Could you check a few things on this model? Use its own coordinates, in mm. Coordinates: 2 decimals unless noted, no trailing zeros. Loops run counter-clockwise (first coordinate to the right, second up) from the corner with the lowest first, then second, coordinate; pieces in that order, holes last.
1) Imagine slicing it at A-A on y = -1. Please give me the cut outline in (x, z).
2) Will these pins go through, and if not, where does the flat tip stop? P1, Ø1, axis at x = -28, y = -2.5, coming from the +Z side; P2, Ø1.5, axis at y = -1.5, z = 35.5, coming from the -X side; P3, Ø1, axis at x = -58.5, y = -1, coming from the +Z side.
3) Imagine slicing it at B-B on x = 12.5. Please give me the cut outline in (y, z).
4) If I drill on line 1 along X through (y, z) = (-2.7, 20); line 2 along Z through (x, y) = (19.5, -0.3); line 3 along X through (y, z) = (-2.1, 27.5), over which ranges is the centre line in solid material (lowest first)?
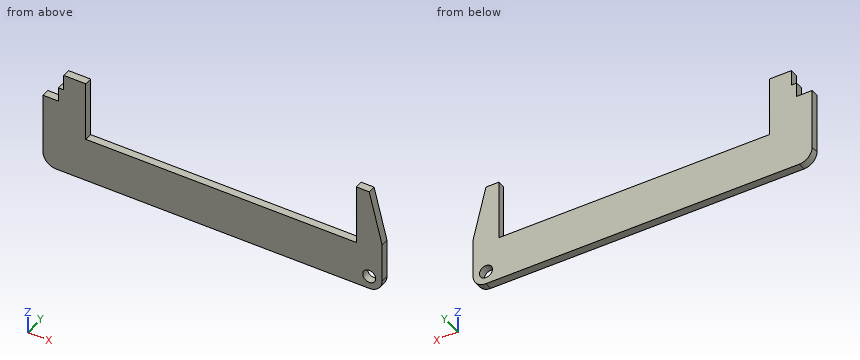
```python
from build123d import *

# Parameters (mm, degrees)
F0_R     = 2.5
F1_DEPTH = 3
F2_W     = 2
F2_H     = 6
F3_DEPTH = 3.001


with BuildPart() as f1:
    # F0 (on Front) → F1 (new body)
    with BuildSketch(Plane.XZ):
        with BuildLine():
            Line((-59.771481, 28.5), (-65.771481, 28.5))
            Line((-65.771481, 28.5), (-65.771481, 5))
            ThreePointArc((-65.771481, 5), (-64.307015, 1.464466), (-60.771481, 0))
            Line((-60.771481, 0), (60.228519, 0))
            ThreePointArc((60.228519, 0), (63.764053, 1.464466), (65.228519, 5))
            Line((65.228519, 5), (65.228519, 20))
            Line((65.228519, 20), (60.228519, 40))
            Line((60.228519, 40), (55.228519, 40))
            Line((55.228519, 40), (55.228519, 17))
            Line((55.228519, 17), (-49.271481, 17))
            Line((-49.271481, 17), (-49.271481, 40))
            Line((-49.271481, 40), (-59.771481, 40))
            Line((-59.771481, 40), (-59.771481, 28.5))
        make_face()
        with Locations((60.228519, 5)):
            Circle(F0_R, mode=Mode.SUBTRACT)
    extrude(amount=F1_DEPTH)

    # F2 (on face) → F3 (cut, through all)
    with BuildSketch(Plane.XZ.offset(3)):
        with Locations((-58.771481, 37)):
            Rectangle(F2_W, F2_H)
    extrude(amount=-F3_DEPTH, mode=Mode.SUBTRACT)


solid = f1.part
```
Filled in:
1. outline: (-65.77, 5) arc R5 ccw to (-60.77, 0) - (60.23, 0) arc R5 ccw to (65.23, 5) - (65.23, 20) - (60.23, 40) - (55.23, 40) - (55.23, 17) - (-49.27, 17) - (-49.27, 40) - (-57.77, 40) - (-57.77, 34) - (-59.77, 34) - (-59.77, 28.5) - (-65.77, 28.5) - close; hole circle Ø5 at (60.23, 5)
2. P1: stops at z = 17
2. P2: stops at x = -57.77
2. P3: stops at z = 34
3. outline: (-3, 0) - (0, 0) - (0, 17) - (-3, 17) - close
4. line 1: x = -65.77 to -49.27, 55.23 to 65.23
4. line 2: z = 0 to 17
4. line 3: x = -65.77 to -49.27, 55.23 to 63.35
